The figure shows three views and two pictorial views of one solid part (mm, origin at its lowest corner). Answer the questions. Coordinates: 2 decimals unless noted, no trailing zeros. Write each loop counter-clockwise with the first axis right and the second up, starting at its lowest first coordinate (ties: lowest second). Pieces come first, ordered by that corner, then holes. Notation, with made-up numbers: M -18.5,85 L 36.5,85 A16 cw 36.5,90 Z; hole C 41.5,78 d10. An arc over 180 degrees is marked long. Use a Markdown table: item, result. Add a question column.
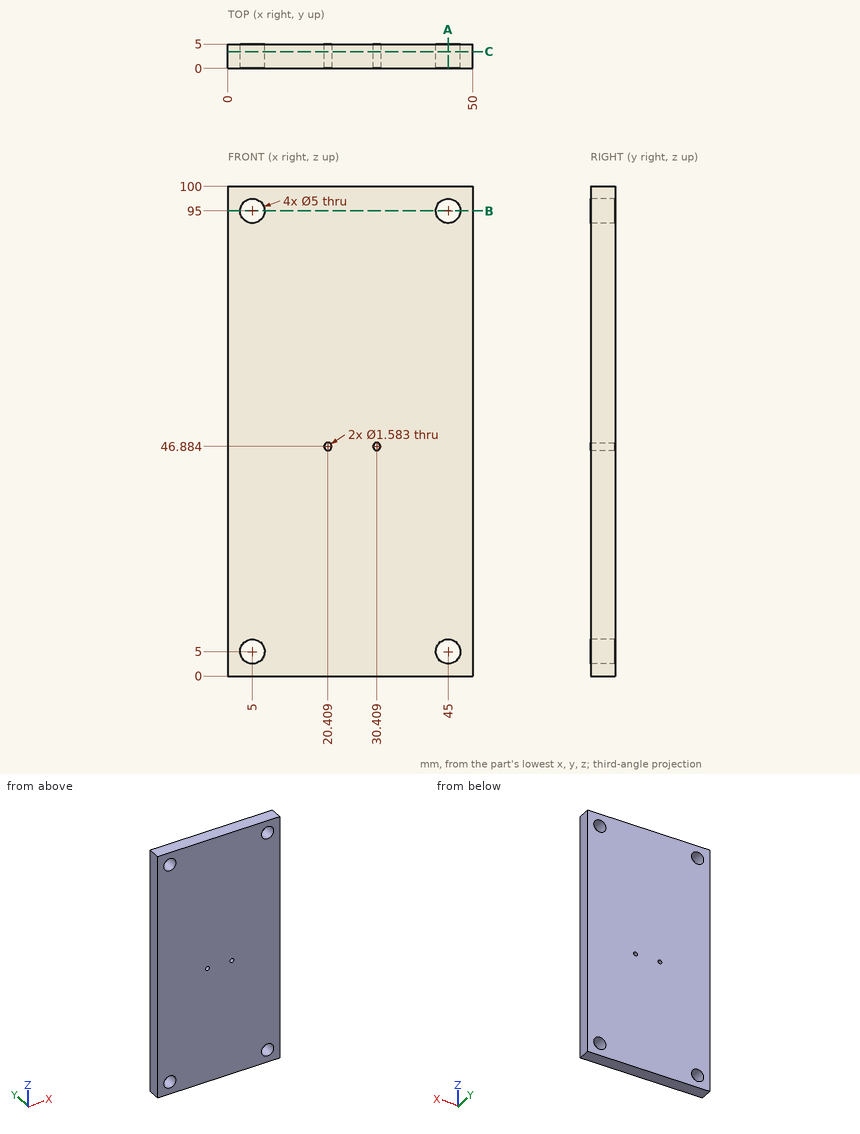
Item 1: This flat-tipped pin is pushed along its axis until it touches: pin 1 (4 mm diameter, centred on x = 5, z = 95, fed in from -Y). Where does it stop, or does it pass through?
Item 2: Consider probe 1 along X at (y, z) = (2.5, 95). Determine where the line is inside the solid, lowest interval first.
Item 3: Find section C-C on y = 3.45. Give the vertices of the cut face in (x, z) (1 decimal).
Item 4: Find section B-B on z = 95. Give the vertices of the cut face in (x, y), then the cut area to 3 significant figures.
Item 5: Find section A-A on x = 45. Give the vertices of the cut face in (y, z), then the cut area to 3 significant figures.
Geometry says:
| question | item | result |
|---|---|---|
| 1 | pin 1 | passes through |
| 2 | probe 1 | x = 0 to 2.5, 7.5 to 42.5, 47.5 to 50 |
| 3 | outline | M 0,0 L 50,0 L 50,100 L 0,100 Z; hole C 5,5 d5; hole C 5,95 d5; hole C 20.4,46.9 d1.6; hole C 30.4,46.9 d1.6; hole C 45,5 d5; hole C 45,95 d5 |
| 4 | outline | M 0,0 L 2.5,0 L 2.5,5 L 0,5 Z; M 7.5,0 L 42.5,0 L 42.5,5 L 7.5,5 Z; M 47.5,0 L 50,0 L 50,5 L 47.5,5 Z |
| 4 | area | 200 mm2 |
| 5 | outline | M 0,0 L 5,0 L 5,2.5 L 0,2.5 Z; M 0,7.5 L 5,7.5 L 5,92.5 L 0,92.5 Z; M 0,97.5 L 5,97.5 L 5,100 L 0,100 Z |
| 5 | area | 450 mm2 |
